The drawing under review shows one solid part. Ordinate dimensions are in mm from its lowest x, y, z. A direction names the side the tool comes from. Round coordinates to 2 decimals unless told otherwise and drop trailing zeros. Order: outer loops, then holes, each group sorted by start corner. A loop starts at its lowest first (then second) coordinate and runs counter-clockwise, first axis right, second up. Notation, with made-up numbers: (37, -20.75) - (53, -20.75) arc R15 ccw to (53, -10.75) - close; hole circle Ø5 at (48, 30). An arc over 180 degrees is marked (long way). One line per question, with ' | ' between items.
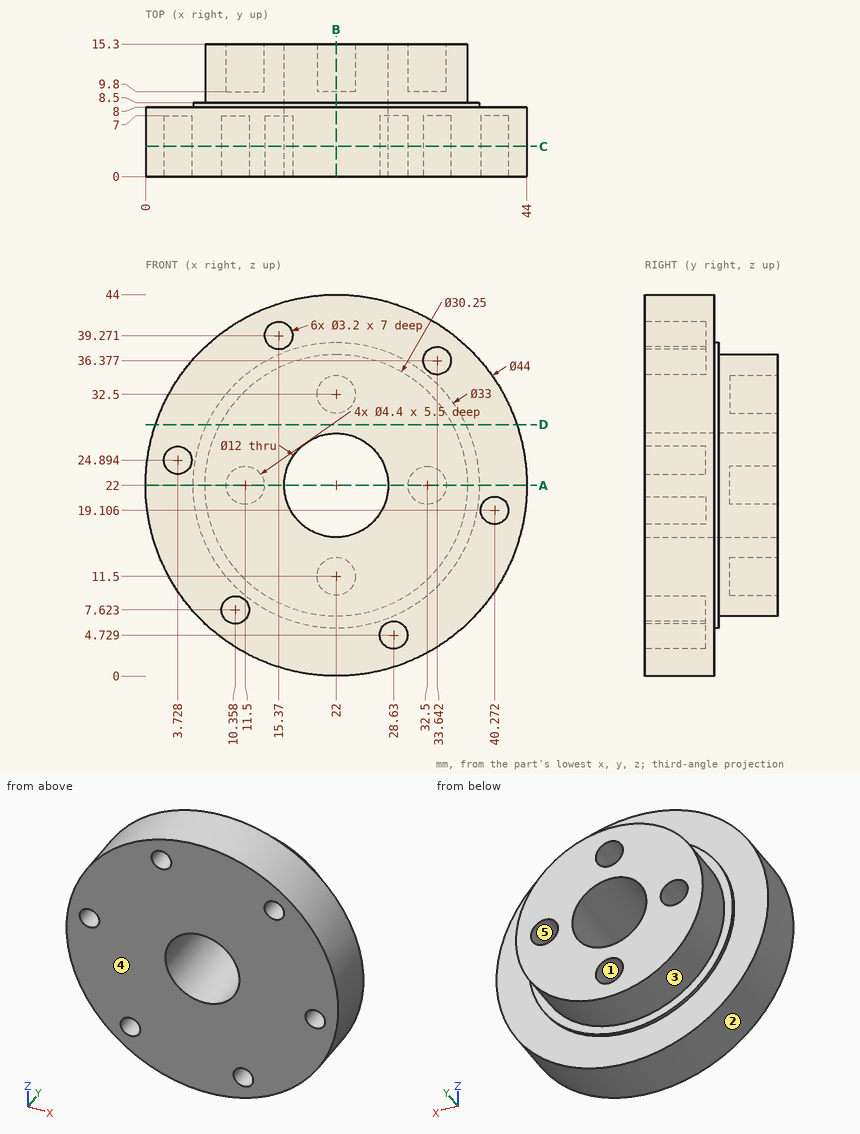
(1) For the marked faces 1 and 2, list the 3-axis set-ups (+Z, -Z, +X, -X, +Y, -Y) from which the entire face can be reached by the end or side of a thin tool; tool diameter is ignored.
Output values:
face 1: +Y | face 2: +Y, -Y
(2) Insertion check: pin 1 (1.3 mm diameter, centred on x = 33, z = 21, fed in from +Y); pin 2 (1 mm diameter, centred on x = 40, z = 19, fed in from -Y); pin 3 (3 mm diameter, centred on x = 40.27, z = 19.11, fed in from +Y). Each pin has a flat end and moves straight along its axis. Give the tip position at first contact, or say it passes through.
Output values:
pin 1: y = 9.8 | pin 2: y = 7 | pin 3: y = 8
(3) We need section B-B on x = 22. State the section outline as (y, z) points (1 decimal).
Output values:
outline: (0, 0) - (8, 0) - (8, 5.5) - (8.5, 5.5) - (8.5, 6.9) - (15.3, 6.9) - (15.3, 9.3) - (9.8, 9.3) - (9.8, 13.7) - (15.3, 13.7) - (15.3, 16) - (0, 16) - close; (0, 28) - (15.3, 28) - (15.3, 30.3) - (9.8, 30.3) - (9.8, 34.7) - (15.3, 34.7) - (15.3, 37.1) - (8.5, 37.1) - (8.5, 38.5) - (8, 38.5) - (8, 44) - (0, 44) - close
(4) We need section D-D on z = 29. State the section outline as (x, y) points.
Output values:
outline: (1.14, 0) - (42.86, 0) - (42.86, 8) - (36.94, 8) - (36.94, 8.5) - (35.41, 8.5) - (35.41, 15.3) - (8.59, 15.3) - (8.59, 8.5) - (7.06, 8.5) - (7.06, 8) - (1.14, 8) - close
(5) We need section A-A on z = 22. State the section outline as (x, y) points (1 decimal).
Output values:
outline: (0, 0) - (16, 0) - (16, 15.3) - (13.7, 15.3) - (13.7, 9.8) - (9.3, 9.8) - (9.3, 15.3) - (6.9, 15.3) - (6.9, 8.5) - (5.5, 8.5) - (5.5, 8) - (0, 8) - close; (28, 0) - (44, 0) - (44, 8) - (38.5, 8) - (38.5, 8.5) - (37.1, 8.5) - (37.1, 15.3) - (34.7, 15.3) - (34.7, 9.8) - (30.3, 9.8) - (30.3, 15.3) - (28, 15.3) - close
(6) For probe 1 along X at (y, z) = (11.4, 22) (1 decimal); probe 2 along X at (y, z) = (2.75, 19) (1 decimal); probe 3 along X at (y, z) = (6, 18) (1 decimal), list the stretches that pass through material, from the lowest coordinate up. Write a range as [from, to].
Output values:
probe 1: [6.9, 9.3], [13.7, 16], [28, 30.3], [34.7, 37.1] | probe 2: [0.2, 16.8], [27.2, 38.7], [41.9, 43.8] | probe 3: [0.4, 17.5], [26.5, 39.1], [41.4, 43.6]
(7) Mouldability with a two-part tool opening along X and no side actions: class the marked faces 3, 4 and 5 as released by +X, released by -X, zero draft, split by the parting line, or undercut.
Output values:
face 3: split by the parting line | face 4: zero draft | face 5: undercut
(8) We need section C-C on y = 3.5. State the section outline as (x, z) points (1 decimal).
Output values:
outline: circle Ø44 at (22, 22); hole circle Ø3.2 at (3.7, 24.9); hole circle Ø3.2 at (10.4, 7.6); hole circle Ø3.2 at (15.4, 39.3); hole circle Ø12 at (22, 22); hole circle Ø3.2 at (28.6, 4.7); hole circle Ø3.2 at (33.6, 36.4); hole circle Ø3.2 at (40.3, 19.1)
